from build123d import *

# Parameters (mm, degrees)
BOSS_EXTRUDE1_DEPTH            = 15
SKETCH3_W                      = 14.708741574
SKETCH3_H                      = 3
CUT_EXTRUDE1_DEPTH             = 50.497474683
M5_CLEARANCE_HOLE1_D           = 5.5
M5_CLEARANCE_HOLE1_CSINK_D     = 5.55
M5_CLEARANCE_HOLE1_CSINK_ANGLE = 90
FILLET1_R                      = 10
CUT_EXTRUDE2_DEPTH             = 60.179810901


with BuildPart() as part:
    # Sketch2 → Boss-Extrude1 (new body)
    with BuildSketch(Plane.XY):
        with BuildLine():
            Line((-25, 40), (-25, 0))
            ThreePointArc((-25, 0), (0, 25), (25, 0))
            Line((25, 0), (25, 40))
            Line((25, 40), (-25, 40))
        make_face()
        with BuildLine():
            ThreePointArc((25, 0), (0, 25), (-25, 0))
            Line((-25, 0), (-10.4, 0))
            ThreePointArc((-10.4, 0), (0, 10.4), (10.4, 0))
            Line((10.4, 0), (25, 0))
        make_face()
        with BuildLine():
            Line((-10.4, 0), (-25, 0))
            ThreePointArc((-25, 0), (0, -25), (25, 0))
            Line((25, 0), (10.4, 0))
            ThreePointArc((10.4, 0), (0, -10.4), (-10.4, 0))
        make_face()
    extrude(amount=BOSS_EXTRUDE1_DEPTH)

    # Sketch3 → Cut-Extrude1 (cut, through all)
    with BuildSketch(Plane.XY.offset(15)):
        with Locations((-17.645629213, 0)):
            Rectangle(SKETCH3_W, SKETCH3_H)
    extrude(amount=-CUT_EXTRUDE1_DEPTH, mode=Mode.SUBTRACT)

    # Sketch10 → CBORE for M5 SHCS3 (revolve, cut)
    with BuildSketch(Plane(origin=(-17.623108927, 40, 7.5), x_dir=(0, 0, 1), z_dir=(1, 0, 0))):
        Polygon((0, 0), (0, 65), (2.75, 65), (2.75, 10), (5, 10), (5, 0.025), (5.025, 0), align=None)
    revolve(axis=Axis((-17.623108927, 46.35, 7.5), (0, -1, 0)), mode=Mode.SUBTRACT)

    # M5 Clearance Hole1 (through all)
    with Locations(Plane.XY.offset(15)):
        with Locations((-7.5, 30), (7.5, 30)):
            CounterSinkHole(M5_CLEARANCE_HOLE1_D / 2, M5_CLEARANCE_HOLE1_CSINK_D / 2, counter_sink_angle=M5_CLEARANCE_HOLE1_CSINK_ANGLE)

    # Fillet1
    # the kernel refuses this fillet: 10 mm, written as the material it takes off along each edge
    with BuildSketch(Plane(origin=(-25, 40, -25), x_dir=(0, -1, 0), z_dir=(0, 0, 1))) as fillet1_piece_1:
        with BuildLine():
            CenterArc((FILLET1_R, FILLET1_R), FILLET1_R, 180, 90)
            Line((0, FILLET1_R), (0, 0))
            Line((0, 0), (FILLET1_R, 0))
        make_face()
    extrude(amount=65, mode=Mode.SUBTRACT)
    with BuildSketch(Plane(origin=(25, 40, -25), x_dir=(0, -1, 0), z_dir=(0, 0, 1))) as fillet1_piece_2:
        with BuildLine():
            CenterArc((FILLET1_R, -FILLET1_R), FILLET1_R, 90, 90)
            Line((0, -FILLET1_R), (0, 0))
            Line((0, 0), (FILLET1_R, 0))
        make_face()
    extrude(amount=65, mode=Mode.SUBTRACT)

    # Sketch18 → Cut-Extrude2 (cut, through all)
    with BuildSketch(Plane(origin=(0, -11.5, 0), x_dir=(1, 0, 0), z_dir=(0, 1, 0))):
        Polygon((-19.99024503, -3.4), (-15.255972823, -3.4), (-12.888836719, -7.5), (-15.255972823, -11.6), (-19.99024503, -11.6), (-22.357381134, -7.5), align=None)
    extrude(amount=-CUT_EXTRUDE2_DEPTH, mode=Mode.SUBTRACT)


solid = part.part
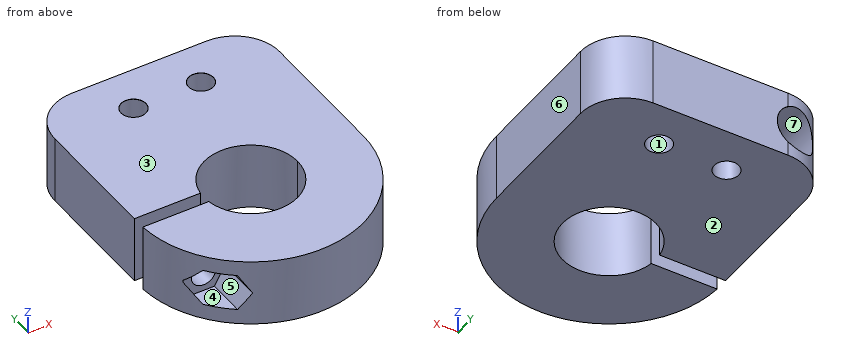
Geometry: final body of the model. Coordinates: model frame, mm. Face numbers are marked on the shaded views. A direction names the side the tool comes from. Coordinates: 2 decimals unless noted, no trailing zeros. Loops run counter-clockwise (first coordinate to the right, second up) from the corner with the lowest first, then second, coordinate; pieces in that order, holes last. Notation, with made-up numbers: (13, 70.5) - (56, 70.5) arc R30 ccw to (56, 104.5) - close; hole circle Ø9 at (4.25, 48). An arc over 180 degrees is marked (long way). Put each result on its own line as item: value. Start each with the question number.
Q1. Line query: line 1 (X direction, y = 15.75, z = 7.5); line 2 (Y direction, x = -14, z = 8.75); line 3 (Y direction, x = -7, z = 2.5). Output: solid intervals per line, ascending.
Q2. Cut plane D-D, the plane z = 9.25. Give the number of separate pieces and of enclosed holes in the cut face, and give its area (3 significant figures).
Q3. Cut plane B-B, the plane y = 9. Return loops of the section in (x, z), and give its area (3 significant figures).
Q4. Set-up query: the marked faces 5, 6 and 7. Return all of +Z, -Z, +X, -X, +Y, -Y with unobstructed straight access to the full face (end or side cutting, diameter ignored); none if empty.
Q5. Pull-direction query (Z, two-part tool) for the marked faces 1, 2, 3 and 4; classes: released by +Z, released by -Z, zero draft, split by the parting line, or undercut.
Q6. Cut plane C-C, the plane y = 22.5. Return loops of the section in (x, z), and give its area (3 significant figures).
Q7. Cut plane A-A, the plane x = 0. Return loops of the section in (y, z), and give its area (3 significant figures).
Q8. Pin query (flat end, axial travel): pin 1 Ø3 at (y, z) = (-3.5, 2) entering from -X; pin 2 Ø8 at (x, z) = (-20, 7.5) entering from +Y; pin 3 Ø6.5 at (x, z) = (-17.62, 7.5) entering from +Y. Return the tip coordinate at first contact, or that it passes through.
Filled sheet:
1. line 1: -25 to -20.37, -14.87 to 25
1. line 2: -11.5 to -1.5, 1.5 to 30
1. line 3: -24 to -7.69, 7.69 to 27.3, 32.7 to 40
2. separate pieces: 3
2. enclosed holes: 2
2. area: 2,210 mm²
3. outline: (-25, 0) - (-5.21, 0) - (-5.21, 15) - (-25, 15) - close; (5.21, 0) - (25, 0) - (25, 15) - (5.21, 15) - close; hole circle Ø5.5 at (-17.62, 7.5)
3. area: 570 mm²
4. face 5: -Y
4. face 6: +Z, -Z, +X, +Y, -Y
4. face 7: +Y
5. face 1: zero draft
5. face 2: released by -Z
5. face 3: released by +Z
5. face 4: undercut
6. outline: (-25, 0) - (25, 0) - (25, 15) - (-25, 15) - close; hole circle Ø5.5 at (-17.62, 7.5)
6. area: 726 mm²
7. outline: (-25, 0) - (-10.4, 0) - (-10.4, 15) - (-25, 15) - close; (10.4, 0) - (40, 0) - (40, 15) - (10.4, 15) - close
7. area: 663 mm²
8. pin 1: x = -24.92
8. pin 2: y = 38.21
8. pin 3: y = 30
